Can you work these out from the model? Positions are in its coordinate system, mm. Face numbers are marked on the shaded views. A direction names the side the tool comes from. Give positions to 0.01 mm unless a question says otherwise; leave off trailing zeros. Loops run counter-clockwise (first coordinate to the right, second up) from the corner with the lowest first, then second, coordinate; pieces in that order, holes last.
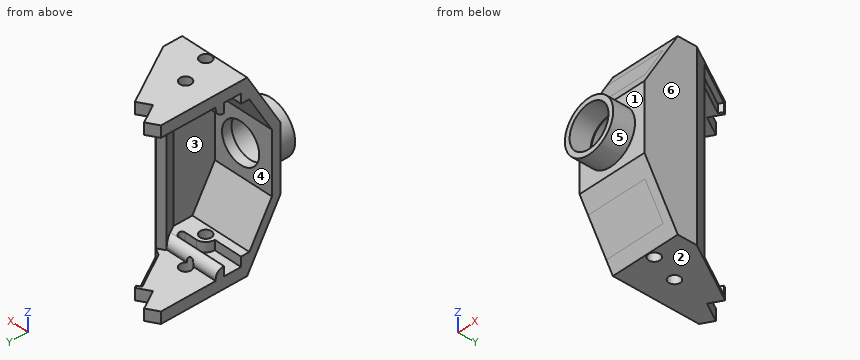
from build123d import *

# Parameters (mm, degrees)
EXTRUDE_1_DEPTH         = 18.35
CUT_EXTRUDE_1_DEPTH     = 95.3
SHELL1_START            = -41.65
SHELL1_DEPTH            = 83.3
SHELL1_START_2          = -18.35
SHELL1_2_DEPTH          = 32.2
CUT_EXTRUDE_2_REACH     = 121.678
SKETCH_5_R              = 13.65
EXTRUDE_2_DEPTH         = 11.5
CUT_EXTRUDE1_DEPTH      = 92.3
SKETCH4_W               = 83.3
SKETCH4_H               = 26.8
CUT_EXTRUDE2_DEPTH      = 4.5
M24_TAPPED_HOLE2_D      = 21
M24_TAPPED_HOLE2_DEPTH  = 16
M24_TAPPED_HOLE2_TIP    = 6.3090365
HOLEWZD2_D              = 22
HOLEWZD2_DEPTH          = 11
SKETCH20_W              = 14.821429848
SKETCH20_H              = 1.5
SKETCH20_W_2            = 17.378570152
BOSS_EXTRUDE2_DEPTH     = 5
FILLET1_R               = 1.5
FILLET2_R               = 4
SKETCH21_W              = 32.2
SKETCH21_H              = 2.401923789
BOSS_EXTRUDE3_DEPTH     = 2
FILLET1_OF_MIRROR1_R    = 1.5
FILLET2_OF_MIRROR1_R    = 4
CUT_EXTRUDE3_DEPTH      = 113.771632022
CUT_EXTRUDE3_DEPTH_BACK = 113.771632022
SKETCH22_R              = 3
FILLET3_R               = 5
CUT_EXTRUDE4_DEPTH      = 109.855137726
CUT_EXTRUDE4_DEPTH_BACK = 109.855137726
SKETCH23_R              = 3


with BuildPart() as part:
    # Эскиз2 → Бобышка-Вытянуть1 (new, symmetric)
    with BuildSketch(Plane(origin=(0, 0, 0), x_dir=(0, 0, -1), z_dir=(1, 0, 0))):
        Polygon((-17.25, 0), (17.25, 0), (47.65, 17.551448183), (47.65, 87.222990915), (-47.65, 87.222990915), (-47.65, 17.551448183), align=None)
    extrude(amount=EXTRUDE_1_DEPTH, both=True)

    # Эскиз3 → Вырез-Вытянуть1 (cut)
    with BuildSketch(Plane(origin=(0, 0, -47.65), x_dir=(-1, 0, 0), z_dir=(0, 0, -1))):
        Polygon((-18.35, 87.222990915), (-18.35, 27.551448183), (6.1746732, 70.029428205), (18.35, 63), (18.35, 87.222990915), align=None)
    extrude(amount=-CUT_EXTRUDE_1_DEPTH, mode=Mode.SUBTRACT)

    # Shell1: read off the stored shape, not the designer's step
    # Shell1 outline → Shell1 (cut)
    with BuildSketch(Plane.XY.offset(SHELL1_START)):
        Polygon((-18.35, 4.5), (13.85, 4.5), (13.85, 26.345676817), (-10.071787517, 67.779428205), (-18.35, 63), align=None)
    extrude(amount=SHELL1_DEPTH, mode=Mode.SUBTRACT)

    # Shell1 2 outline → Shell1 2 (add)
    with BuildSketch(Plane.YZ.offset(SHELL1_START_2)):
        Polygon((19.283498991, -41.65), (4.5, -16.044228634), (4.5, -25.044228634), (14.087346568, -41.65), align=None)
        Polygon((14.087346568, 41.65), (4.5, 25.044228634), (4.5, 16.044228634), (19.283498991, 41.65), align=None)
    extrude(amount=SHELL1_2_DEPTH)

    # Вырез-Вытянуть2: up to this face of the body (flat: up to its plane)
    cut_extrude_2_end = Plane(part.part.faces().sort_by_distance((-3.441629471, 38.42100508, 47.65))[0])
    # Эскиз4 → Вырез-Вытянуть2 (cut, up to the picked face)
    with BuildSketch(Plane(origin=(0, 0, -47.65), x_dir=(-1, 0, 0), z_dir=(0, 0, -1)), mode=Mode.PRIVATE) as cut_extrude_2_sk1:
        Polygon((6.1746732, 70.029428205), (12.496658648, 66.379428205), (6.646658648, 56.246930981), (0.3246732, 59.896930981), align=None)
    cut_extrude_2_tool1 = split(extrude(cut_extrude_2_sk1.sketch, amount=-CUT_EXTRUDE_2_REACH, mode=Mode.PRIVATE), bisect_by=cut_extrude_2_end, keep=Keep.BOTH, mode=Mode.PRIVATE)
    add(cut_extrude_2_tool1.solids().sort_by(Axis((-6.410666, 63.13818, -47.65), (0, 0, 1)))[0], mode=Mode.SUBTRACT)

    # Эскиз5 → Бобышка-Вытянуть2 (add)
    with BuildSketch(Plane.XZ):
        with Locations(Location((-0.65, 0, 0), (0, 0, 270))):
            Circle(SKETCH_5_R)
    extrude(amount=EXTRUDE_2_DEPTH)

    # Sketch3 → Cut-Extrude1 (cut)
    with BuildSketch(Plane.XY.offset(46.15)):
        Polygon((13.35, 36.211702221), (0.4253268, 58.597892875), (-1.73973671, 57.347892875), (9.019872981, 38.711702221), align=None)
    extrude(amount=-CUT_EXTRUDE1_DEPTH, mode=Mode.SUBTRACT)

    # Sketch4 → Cut-Extrude2 (cut)
    with BuildSketch(Plane(origin=(25.692627019, 14.833645126, 0), x_dir=(0, 0, -1), z_dir=(0.8660254037844454, 0.4999999999999885, 0))):
        with Locations((0, 38.634600438)):
            Rectangle(SKETCH4_W, SKETCH4_H)
    extrude(amount=-CUT_EXTRUDE2_DEPTH, mode=Mode.SUBTRACT)

    # M24 Tapped Hole2
    with Locations(Plane(origin=(0, -11.5, 0), x_dir=(-1, 0, 0), z_dir=(0, -1, 0))):
        with Locations((0.65, 0)):
            Hole(M24_TAPPED_HOLE2_D / 2, depth=M24_TAPPED_HOLE2_DEPTH)
            with Locations((0, 0, -(M24_TAPPED_HOLE2_DEPTH + M24_TAPPED_HOLE2_TIP / 2))):  # 118° drill point
                Cone(0, M24_TAPPED_HOLE2_D / 2, M24_TAPPED_HOLE2_TIP, mode=Mode.SUBTRACT)

    # HoleWzd2
    with Locations(Plane(origin=(-0.65, -11.5, 0), x_dir=(0, 0, -1), z_dir=(0, -1, 0))):
        with Locations((0, 0)):
            Hole(HOLEWZD2_D / 2, depth=HOLEWZD2_DEPTH)

    # Sketch20 → Boss-Extrude2 (add)
    with BuildSketch(Plane.XY.offset(-41.65)):
        with Locations((-10.939285076, 18.533498991)):
            Rectangle(SKETCH20_W, SKETCH20_H)
        with Locations((-10.939285076, 20.033498991)):
            Rectangle(SKETCH20_W, SKETCH20_H)
        Polygon((-3.528570152, 25.891773598), (-3.528570152, 20.783498991), (13.85, 20.783498991), (13.85, 25.891773598), (10.503833111, 25.891773598), align=None)
        Polygon((11.860101568, 29.792282004), (8.251873533, 29.792282004), (10.503833111, 25.891773598), (13.85, 25.891773598), (13.85, 26.345676817), align=None)
        Polygon((-18.35, 34.110173911), (-18.35, 29.792282004), (8.251873533, 29.792282004), (11.860101568, 29.792282004), (9.367165513, 34.110173911), align=None)
        with Locations((5.160714924, 18.533498991)):
            Rectangle(SKETCH20_W_2, SKETCH20_H)
        with Locations((5.160714924, 20.033498991)):
            Rectangle(SKETCH20_W_2, SKETCH20_H)
    boss_extrude2 = extrude(amount=BOSS_EXTRUDE2_DEPTH)

    # Fillet1
    fillet1_edges = [part.edges().sort_by_distance(p)[0] for p in [
        (10.503833111, 25.891773598, -39.15),
        (8.251873533, 29.792282004, -39.15),
    ]]
    fillet(fillet1_edges, radius=FILLET1_R)

    # Fillet2
    fillet2_edges = [part.edges().sort_by_distance(p)[0] for p in [
        (-4.491417244, 34.110173911, -36.65),
    ]]
    fillet(fillet2_edges, radius=FILLET2_R)

    # Sketch21 → Boss-Extrude3 (add)
    with BuildSketch(Plane.XZ.offset(-17.783498991)):
        with Locations((-2.25, -37.850961895)):
            Rectangle(SKETCH21_W, SKETCH21_H)
    boss_extrude3 = extrude(amount=BOSS_EXTRUDE3_DEPTH)

    # Mirror1: Boss-Extrude2, Boss-Extrude3 across plane
    add(boss_extrude2.mirror(Plane.XY))
    add(boss_extrude3.mirror(Plane.XY))

    # Fillet1 of Mirror1
    fillet1_of_mirror1_edges = [part.edges().sort_by_distance(p)[0] for p in [
        (10.503833111, 25.891773598, 39.15),
        (8.251873533, 29.792282004, 39.15),
    ]]
    fillet(fillet1_of_mirror1_edges, radius=FILLET1_OF_MIRROR1_R)

    # Fillet2 of Mirror1
    fillet2_of_mirror1_edges = [part.edges().sort_by_distance(p)[0] for p in [
        (-4.491417244, 34.110173911, 36.65),
    ]]
    fillet(fillet2_of_mirror1_edges, radius=FILLET2_OF_MIRROR1_R)

    # Sketch22 → Cut-Extrude3 (cut, two sides: drawn at the far end of the back side and taken through both)
    with BuildSketch(Plane.XY.offset(-41.65).offset(-CUT_EXTRUDE3_DEPTH_BACK)):
        with Locations((-3.85, 36.499622644)):
            Circle(SKETCH22_R)
    extrude(amount=CUT_EXTRUDE3_DEPTH + CUT_EXTRUDE3_DEPTH_BACK, mode=Mode.SUBTRACT)

    # Fillet3
    fillet3_edges = [part.edges().sort_by_distance(p)[0] for p in [
        (-3.528570152, 25.891773598, -39.15),
    ]]
    fillet(fillet3_edges, radius=FILLET3_R)

    # Sketch23 → Cut-Extrude4 (cut, two sides: drawn at the far end of the back side and taken through both)
    with BuildSketch(Plane.XY.offset(-36.65).offset(-CUT_EXTRUDE4_DEPTH_BACK)):
        with Locations((1.471429848, 20.891773598)):
            Circle(SKETCH23_R)
    extrude(amount=CUT_EXTRUDE4_DEPTH + CUT_EXTRUDE4_DEPTH_BACK, mode=Mode.SUBTRACT)


solid = part.part
(1) Suppose I cut it at D-D on y = 10. List the corners of the cut face in (x, z) for me.
Returned:
outline: (-18.35, -34.57) - (18.35, -34.57) - (18.35, 34.57) - (-18.35, 34.57) - (-18.35, 25.57) - (13.85, 25.57) - (13.85, -25.57) - (-18.35, -25.57) - close
(2) Suppose I cut it at C-C on y = 32. List the corners of the cut face in (x, z) for me, plus the area to 3 significant figures.
Returned:
outline: (-18.35, -47.65) - (15.78, -47.65) - (15.78, 47.65) - (-18.35, 47.65) - (-18.35, 37.12) - (10.59, 37.12) - (10.59, -37.12) - (-18.35, -37.12) - close
area: 1,100 mm2
(3) Will these pins go through, and if not, where does the flat tip stop? P1, Ø2, axis at x = -3.5, y = 14, coming from the +Z side; P2, Ø8, axis at x = 11.5, y = 7.5, coming from the -Z side; P3, Ø10, axis at x = -14.5, y = 10, coming from the -Z side.
Returned:
P1: stops at z = 43.23
P2: stops at z = -37.17
P3: stops at z = -43.23
(4) Which directions (+Z, -Z, +X, -X, +Y, -Y) give clear straight access to the entire face, cutting with the end or side of a thin tool? Please do the marked faces 4, 5 and 6.
Returned:
face 4: -X
face 5: -Y
face 6: +Z, -Z, +X, +Y, -Y
(5) Suppose I cut it at B-B on y = 53. List the corners of the cut face in (x, z) for me, plus the area to 3 significant figures.
Returned:
outline: (-18.35, -47.65) - (3.66, -47.65) - (3.66, -46.15) - (0.77, -46.15) - (0.77, -41.65) - (-18.35, -41.65) - close; (-18.35, 41.65) - (0.77, 41.65) - (0.77, 46.15) - (3.66, 46.15) - (3.66, 47.65) - (-18.35, 47.65) - close
area: 238 mm2
(6) Please list where these lines run through material, in increasing order: probe 1 along Z at (x, y) = (-8, 45); probe 2 along X at (y, z) = (21.5, 8.5).
Returned:
probe 1: z = -47.65 to -41.65, 41.65 to 47.65
probe 2: x = 13.85 to 18.35
(7) Suppose I cut it at A-A on z = 0. List the corners of the cut face in (x, y) for me.
Returned:
outline: (-18.35, 0) - (-14.3, 0) - (-14.3, -11.5) - (-11.65, -11.5) - (-11.65, -0.5) - (-11.15, -0.5) - (-11.15, 4.5) - (-18.35, 4.5) - close; (9.18, 34.44) - (13.85, 26.35) - (13.85, 4.5) - (9.85, 4.5) - (9.85, -0.5) - (10.35, -0.5) - (10.35, -11.5) - (13, -11.5) - (13, 0) - (18.35, 0) - (18.35, 27.55) - (13.35, 36.21) - (12.8, 36.53) - close
(8) Thinking about a two-plate mould opening in Y: for the marked faces 1, 2 and 3, which applies, pulls with the +Y half, pulls with the -Y half, needs draft (parallel to the pull), parting line crosses it, or undercut?
Returned:
face 1: pulls with the -Y half
face 2: needs draft
face 3: undercut
